Autodesk Inventor part; units mm, degrees
ref_plane "YZ Plane" through (0, 0, 0) normal (1, 0, 0) x (0, 1, 0)
ref_plane "XZ Plane" through (0, 0, 0) normal (0, 1, 0) x (-1, 0, 0)
ref_plane "XY Plane" through (0, 0, 0) normal (0, 0, 1) x (1, 0, 0)
sketch "main" plane through (0, 0, 0) normal (0, 0, 1) x (1, 0, 0)
  circle A0 centre (-8.7196, -23.7408) radius 2.0955
  circle A1 centre (-34.1196, -23.7408) radius 2.0955
  arc A2 (-34.1196, -17.3908) -> (-34.1196, -30.0908) centre (-34.1196, -23.7408) ccw
  arc A3 (-16.1491, -17.3908) -> (-6.6241, -7.8658) centre (-16.1491, -7.8658) ccw
  arc A4 (-8.7196, -30.0908) -> (-3.6396, -27.5508) centre (-8.7196, -23.7408) ccw
  line L0 (-16.1491, -17.3908) -> (-34.1196, -17.3908)
  line L1 (-8.7196, -30.0908) -> (-34.1196, -30.0908)
  circle A5 centre (-8.7196, 27.0592) radius 2.0955
  circle A6 centre (-34.1196, 27.0592) radius 2.0955
  arc A7 (-34.1196, 33.4092) -> (-34.1196, 20.7092) centre (-34.1196, 27.0592) ccw
  line L2 (-6.6241, 14.3592) -> (-6.6241, -7.8658)
  line L3 (-34.1196, 20.7092) -> (-12.9741, 20.7092)
  arc A8 (-6.6241, 14.3592) -> (-12.9741, 20.7092) centre (-12.9741, 14.3592) ccw
  line L4 (-3.6396, -27.5508) -> (34.4604, 23.2492)
  line L5 (-34.1196, 33.4092) -> (29.3804, 33.4092)
  line L6 (-6.6241, 20.7092) -> (15.6009, 20.7092) construction
  circle A9 centre (3.9804, 27.0592) radius 2.0955
  circle A10 centre (29.3804, 27.0592) radius 2.0955
  arc A11 (34.4604, 23.2492) -> (29.3804, 33.4092) centre (29.3804, 27.0592) ccw
  point P0 (-9.3122, 5.0882)
  dimension "d0" = 4.191
  dimension "d1" = 4.191
  dimension "d2" = 4.191
  dimension "d3" = 4.191
  dimension "d4" = 9.525
  dimension "d5" = 6.35
sketch "Sketch1" plane through (0, 0, 0) normal (0, 0, 1) x (1, 0, 0)
  circle A0 centre (25.4, 0) radius 2.0955
  circle A1 centre (0, 0) radius 2.0955
  arc A2 (0, 6.35) -> (0, -6.35) centre (0, 0) ccw
  arc A3 (17.9705, 6.35) -> (27.4955, 15.875) centre (17.9705, 15.875) ccw
  arc A4 (25.4, -6.35) -> (30.48, -3.81) centre (25.4, 0) ccw
  line L0 (17.9705, 6.35) -> (0, 6.35)
  line L1 (25.4, -6.35) -> (0, -6.35)
  circle A5 centre (25.4, 50.8) radius 2.0955
  circle A6 centre (0, 50.8) radius 2.0955
  arc A7 (0, 57.15) -> (0, 44.45) centre (0, 50.8) ccw
  line L2 (27.4955, 38.1) -> (27.4955, 15.875)
  line L3 (0, 44.45) -> (21.1455, 44.45)
  arc A8 (27.4955, 38.1) -> (21.1455, 44.45) centre (21.1455, 38.1) ccw
  line L4 (30.48, -3.81) -> (68.58, 46.99)
  line L5 (0, 57.15) -> (63.5, 57.15)
  line L6 (27.4955, 44.45) -> (49.7205, 44.45) construction
  circle A9 centre (38.1, 50.8) radius 2.0955
  circle A10 centre (63.5, 50.8) radius 2.0955
  arc A11 (68.58, 46.99) -> (63.5, 57.15) centre (63.5, 50.8) ccw
extrude "Extrusion1" add sketch "Sketch1" along normal blind 1.5875
properties part number "gusset" material "Acetal Resin, White"
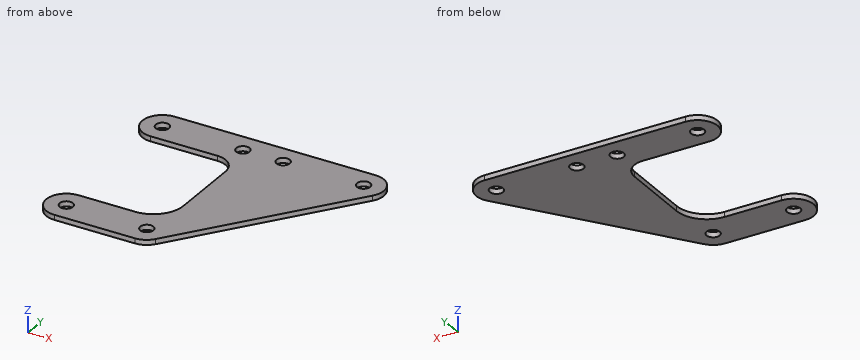
Geometry: final body of the model. Coordinates: model frame, mm. Round coordinates to 2 decimals unless told otherwise and drop trailing zeros. Order: outer loops, then holes, each group sorted by start corner. A loop starts at its lowest first (then second) coordinate and runs counter-clockwise, first axis right, second up. Notation, with made-up numbers: (-17, -39) -> (-12, -39) arc R21 cw to (-12, -19) -> close; hole circle Ø9 at (-19.75, 72). An arc over 180 degrees is marked (long way). Use CSV: the item, a comma, the result in double quotes. Start each with the question number.
1) Section D-D (y = 0). Return the cut outline in (x, z).
2) First-contact query: pin 1 Ø4 at (x, y) = (10, 3.5) entering from -Z; pin 2 Ø0.5 at (y, z) = (21.5, 1) entering from -X. Flat tips, straight axial feed; report the tip coordinate or a pass-through.
3) Section C-C (z = 0.55). State how many separate pieces and enclosed holes the cut face has, and give its area (3 significant figures).
4) Material intervals for line 1 along Y through (x, z) = (0, 0.9); line 2 along Y through (x, z) = (18.5, 0.5); line 3 along Y through (x, z) = (63.5, 0.5), sorted ascending. Write a range as from..to.
5) Section A-A (y = 50.8). Return the cut outline in (x, z).
6) Section B-B (x = 38.1). Return the cut outline in (y, z).
Returned:
1,outline,"(-6.35, 0) -> (-2.1, 0) -> (-2.1, 1.59) -> (-6.35, 1.59) -> close; (2.1, 0) -> (23.3, 0) -> (23.3, 1.59) -> (2.1, 1.59) -> close; (27.5, 0) -> (33.34, 0) -> (33.34, 1.59) -> (27.5, 1.59) -> close"
2,pin 1,"stops at z = 0"
2,pin 2,"stops at x = 27.5"
3,separate pieces,"1"
3,enclosed holes,"6"
3,area,"2,310 mm²"
4,line 1,"y = -6.35..-2.1, 2.1..6.35, 44.45..48.7, 52.9..57.15"
4,line 2,"y = -6.35..6.36, 44.45..57.15"
4,line 3,"y = 40.22..48.7, 52.9..57.15"
5,outline,"(-6.35, 0) -> (-2.1, 0) -> (-2.1, 1.59) -> (-6.35, 1.59) -> close; (2.1, 0) -> (23.3, 0) -> (23.3, 1.59) -> (2.1, 1.59) -> close; (27.5, 0) -> (36, 0) -> (36, 1.59) -> (27.5, 1.59) -> close; (40.2, 0) -> (61.4, 0) -> (61.4, 1.59) -> (40.2, 1.59) -> close; (65.6, 0) -> (69.85, 0) -> (69.85, 1.59) -> (65.6, 1.59) -> close"
6,outline,"(6.35, 0) -> (48.7, 0) -> (48.7, 1.59) -> (6.35, 1.59) -> close; (52.9, 0) -> (57.15, 0) -> (57.15, 1.59) -> (52.9, 1.59) -> close"
